```python
from build123d import *

# Parameters (mm, degrees)
SKETCH1_W            = 115
SKETCH1_H            = 90
BOSS_EXTRUDE1_DEPTH  = 3
SKETCH2_R            = 6.25
CUT_EXTRUDE1_DEPTH   = 3
LPATTERN1_COUNT      = 4
LPATTERN1_PITCH      = 25
LPATTERN1_COUNT_DIR2 = 3
LPATTERN1_PITCH_DIR2 = 25
FILLET1_R            = 3
M5_CLEARANCE_HOLE1_D = 5.3


with BuildPart() as part:
    # Sketch1 → Boss-Extrude1 (new body)
    with BuildSketch(Plane(origin=(0, 0, 0), x_dir=(1, 0, 0), z_dir=(0, 1, 0))):
        with Locations((57.5, 45)):
            Rectangle(SKETCH1_W, SKETCH1_H)
    extrude(amount=BOSS_EXTRUDE1_DEPTH)

    # Sketch2 → Cut-Extrude1 (cut)
    with BuildSketch(Plane(origin=(0, 3, 0), x_dir=(1, 0, 0), z_dir=(0, 1, 0))):
        with Locations(Location((20, 70, 0), (0, 0, 270))):
            Circle(SKETCH2_R)
    cut_extrude1 = extrude(amount=-CUT_EXTRUDE1_DEPTH, mode=Mode.SUBTRACT)

    # LPattern1: Cut-Extrude1 4 × 3
    with Locations(*[(i * LPATTERN1_PITCH, 0, j * LPATTERN1_PITCH_DIR2) for i in range(LPATTERN1_COUNT) for j in range(LPATTERN1_COUNT_DIR2) if (i, j) != (0, 0)]):
        add(cut_extrude1, mode=Mode.SUBTRACT)

    # Fillet1
    fillet1_edges = [part.edges().sort_by_distance(p)[0] for p in [
        (0, 1.5, -90),
        (115, 1.5, -90),
        (115, 1.5, 0),
        (0, 1.5, 0),
    ]]
    fillet(fillet1_edges, radius=FILLET1_R)

    # M5 Clearance Hole1 (through all)
    with Locations(Plane(origin=(0, 3, 0), x_dir=(1, 0, 0), z_dir=(0, 1, 0))):
        with Locations((5, 85), (5, 5), (110, 5), (110, 85)):
            Hole(M5_CLEARANCE_HOLE1_D / 2)


solid = part.part
```
Here's how the part is built. I have some questions about the finished solid (model axes, mm). Coordinates: 2 decimals unless noted, no trailing zeros. Order: outer loops, then holes, each group sorted by start corner. A loop starts at its lowest first (then second) coordinate and runs counter-clockwise, first axis right, second up. Notation, with made-up numbers: (8, 58) -> (13, 58) arc R9 cw to (13, 70) -> close; hole circle Ø10 at (73, -2.75). An arc over 180 degrees is marked (long way). Return JSON: item names as keys, results as strings.
1) Thinking about a two-plate mould opening in X: for faces 1 (the cylindrical face through (114.1, 1.52, -0.86)), 2 (the flat face through (57, 1, -90)), 3 (the cylindrical face through (0.86, 1.52, -0.9)), 4 (the cylindrical face through (110.57, 1.48, -82.41)), which applies, +X half, -X half, draft (parallel to the pull), parting line (faces both ways), or undercut?
Conclusion:
{"face 1": "+X half", "face 2": "draft", "face 3": "-X half", "face 4": "undercut"}
2) If we section it at A-A on z = -85: List the corners of the cut face in (x, y) for me, plus the area to 3 significant figures.
Conclusion:
{"outline": "(0, 0) -> (2.35, 0) -> (2.35, 3) -> (0, 3) -> close; (7.65, 0) -> (107.35, 0) -> (107.35, 3) -> (7.65, 3) -> close; (112.65, 0) -> (115, 0) -> (115, 3) -> (112.65, 3) -> close", "area": "313 mm²"}
3) If we section it at D-D on z = -21.5: List the corners of the cut face in (x, y) for me, plus the area to 3 significant figures.
Conclusion:
{"outline": "(0, 0) -> (13.93, 0) -> (13.93, 3) -> (0, 3) -> close; (26.07, 0) -> (38.93, 0) -> (38.93, 3) -> (26.07, 3) -> close; (51.07, 0) -> (63.93, 0) -> (63.93, 3) -> (51.07, 3) -> close; (76.07, 0) -> (88.93, 0) -> (88.93, 3) -> (76.07, 3) -> close; (101.07, 0) -> (115, 0) -> (115, 3) -> (101.07, 3) -> close", "area": "199 mm²"}
4) If I drill on probe 1 along Z at (x, y) = (95.5, 0.95); probe 2 along Z at (x, y) = (110, 2.05); probe 3 along X at (y, z) = (2.45, -45), over which ranges is the centre line in solid material (lowest first)?
Conclusion:
{"probe 1": "z = -90 to -76.23, -63.77 to -51.23, -38.77 to -26.23, -13.77 to 0", "probe 2": "z = -90 to -87.65, -82.35 to -7.65, -2.35 to 0", "probe 3": "x = 0 to 13.75, 26.25 to 38.75, 51.25 to 63.75, 76.25 to 88.75, 101.25 to 115"}
5) If we section it at C-C on x = 5: List the corners of the cut face in (y, z) for me.
Conclusion:
{"outline": "(0, -90) -> (3, -90) -> (3, -87.65) -> (0, -87.65) -> close; (0, -82.35) -> (3, -82.35) -> (3, -7.65) -> (0, -7.65) -> close; (0, -2.35) -> (3, -2.35) -> (3, 0) -> (0, 0) -> close"}
6) If we section it at B-B on x = 95: List the corners of the cut face in (y, z) for me.
Conclusion:
{"outline": "(0, -90) -> (3, -90) -> (3, -76.25) -> (0, -76.25) -> close; (0, -63.75) -> (3, -63.75) -> (3, -51.25) -> (0, -51.25) -> close; (0, -38.75) -> (3, -38.75) -> (3, -26.25) -> (0, -26.25) -> close; (0, -13.75) -> (3, -13.75) -> (3, 0) -> (0, 0) -> close"}
